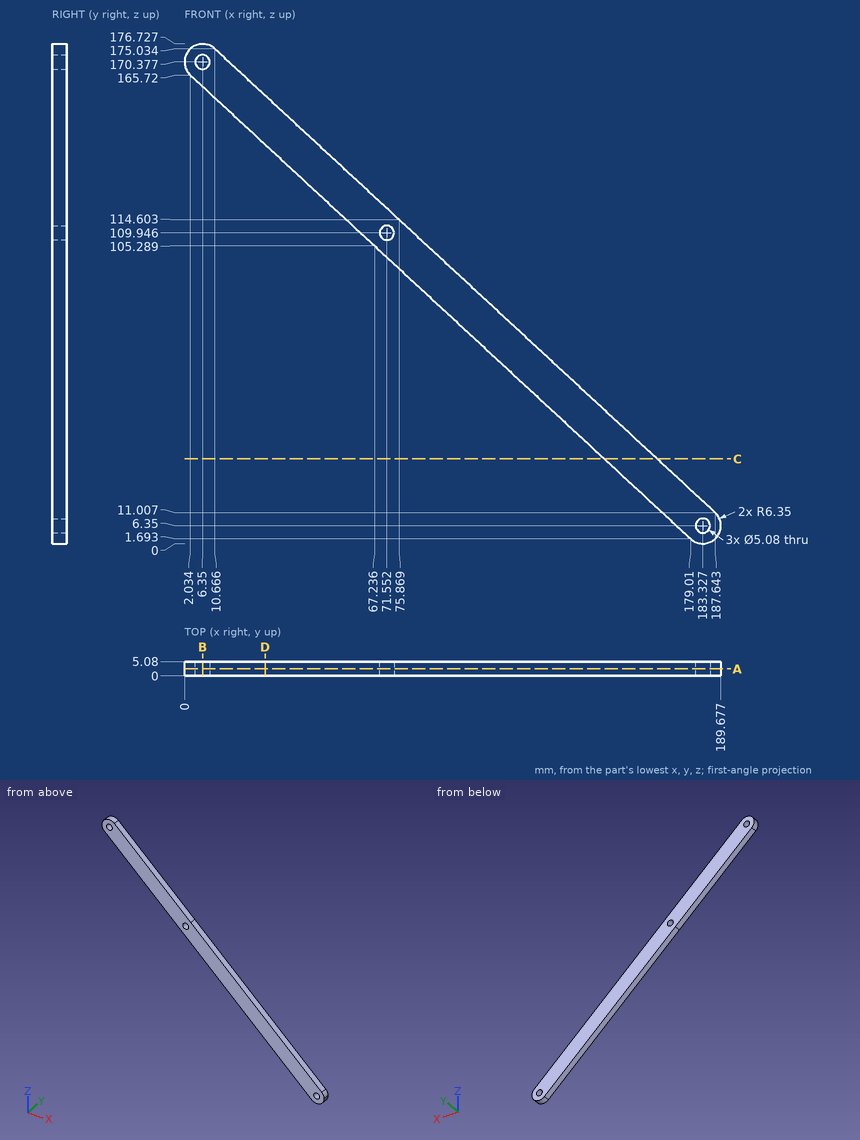
The figure shows three views and two pictorial views of one solid part (mm, origin at its lowest corner). Answer the questions. Give positions to 0.01 mm unless a question says otherwise; leave off trailing zeros. Loops run counter-clockwise (first coordinate to the right, second up) from the corner with the lowest first, then second, coordinate; pieces in that order, holes last. Notation, with made-up numbers: (-27.5, 85.25) -> (-21.5, 85.25) arc R32 cw to (-21.5, 119.25) -> close; hole circle Ø9 at (42.25, -36.75). An arc over 180 degrees is marked (long way). Put each result on its own line as item: value. Start each with the question number.
Item 1: The part is cut by section C-C (z = 30). Give the vertices of the cut face in (x, y).
Item 2: The part is cut by section D-D (x = 28.5). Give the vertices of the cut face in (y, z) (1 decimal).
Item 3: The part is cut by section A-A (y = 2.55). State how many separate pieces and enclosed holes the cut face has, then the cut area to 3 significant figures.
Item 4: Find the intervals of material crossed by L1, parallel to X at y = 1.8, z = 170 (1 decimal); L2, parallel to X at y = 0.2, z = 110.5 (1 decimal); L3, parallel to Z at x = 8, y = 1.15 (1 decimal), in increasing order. Write a range as [from, to].
Item 5: Each of these flat-tipped pins is pushed along its axis until it touches: P1, Ø2, axis at y = 4.5, z = 32.5, coming from the +X side; P2, Ø2, axis at y = 2.5, z = 97, coming from the +X side. Where does it stop, or does it pass through?
Item 6: The part is cut by section B-B (x = 6.35). Give the vertices of the cut face in (y, z).
Answers below:
1. outline: (148.47, 0) -> (167.15, 0) -> (167.15, 5.08) -> (148.47, 5.08) -> close
2. outline: (0, 141.2) -> (5.1, 141.2) -> (5.1, 158.5) -> (0, 158.5) -> close
3. separate pieces: 1
3. enclosed holes: 3
3. area: 3,130 mm2
4. L1: [0, 3.8], [8.9, 16.1]
4. L2: [61.6, 69.1], [74, 80.3]
4. L3: [160.2, 168.4], [172.3, 176.5]
5. P1: x = 165.53
5. P2: x = 95.94
6. outline: (0, 161.72) -> (5.08, 161.72) -> (5.08, 167.84) -> (0, 167.84) -> close; (0, 172.92) -> (5.08, 172.92) -> (5.08, 176.73) -> (0, 176.73) -> close
